from build123d import *

# Parameters (mm, degrees)
F0_W          = 465
F0_H          = 360
F1_DEPTH      = 82
F3_DEPTH      = 238.8411541644
F3_DEPTH_BACK = 251
F5_DEPTH      = 190
F5_DEPTH_BACK = 341
F6_T          = 18
F6_T3_DEPTH   = 370.2074342574
F6_T5_DEPTH   = 471


# Not quite as in the source:
# - a shell that OpenCascade refuses in one call is made with other operations: the cavity is built on its own and cut out


with BuildPart() as f1:
    # F0 (on Top) → F1 (new body)
    with BuildSketch(Plane.XY):
        with Locations((6.3401541644, 0)):
            Rectangle(F0_W, F0_H)
    extrude(amount=-F1_DEPTH)

    # F2 (on Right) → F3 (cut, two sides)
    with BuildSketch(Plane.YZ) as f3_sk:
        Polygon((-210, -15), (-210, -112), (-150, -112), (-167.1037171287, -15), align=None)
        Polygon((210, -15), (167.1037171287, -15), (150, -112), (210, -112), align=None)
    extrude(amount=F3_DEPTH, mode=Mode.SUBTRACT)
    extrude(f3_sk.sketch, amount=-F3_DEPTH_BACK, mode=Mode.SUBTRACT)

    # F4 (on Front) → F5 (cut, two sides)
    with BuildSketch(Plane.XZ) as f5_sk:
        Polygon((-241.1598458356, -15), (-241.1598458356, -185.1384545885), (-181.1598458356, -185.1384545885), (-211.1598458356, -15), align=None)
        Polygon((253.8401541644, -15), (223.8401541644, -15), (193.8816988413, -154.3605614963), (253.8401541644, -156.5929672103), align=None)
    extrude(amount=F5_DEPTH, mode=Mode.SUBTRACT)
    extrude(f5_sk.sketch, amount=-F5_DEPTH_BACK, mode=Mode.SUBTRACT)

    # F6: shell of thickness 18, made by hand


with BuildPart() as f6_core1:
    # F6_t2: copy of F1
    add(f1.part)

    # the walls: a layer under each face that stays
    f6_faces = [f6_core1.faces().sort_by_distance(p)[0] for p in [
        (-226.1598458356, 0, -7.5),
        (6.3401541644, -180, -7.5),
        (238.8401541644, 0, -7.5),
        (223.3401541644, 168, -15),
        (6.3401541644, 161.196763275, -48.5),
        (5.0455852734, 0, -82),
        (216.6386314197, 0, -48.5),
        (6.3401541644, -161.196763275, -48.5),
        (-205.2528919819, 0, -48.5),
        (6.3401541644, 180, -7.5),
    ]]
    thicken(f6_faces, amount=-F6_T, mode=Mode.SUBTRACT)

    # F6_s4 → F6_t3 (cut)
    with BuildSketch(Plane.XZ.offset(-185.1037171287)):
        Polygon((-211.3371112312, -15.211256672), (-211.1598458356, 3), (-196.0560524744, 3), (-193.4333062814, -11.874332802), align=None)
        Polygon((224.0161338598, -15.2178305009), (223.8401541644, 3), (209.2984141185, 3), (206.2421846213, -11.2169499127), align=None)
    extrude(amount=F6_T3_DEPTH, mode=Mode.SUBTRACT)

    # F6_s6 → F6_t5 (cut)
    with BuildSketch(Plane.YZ.offset(-229.1598458356)):
        Polygon((-167.2809825243, -15.211256672), (-167.1037171287, 3), (-151.9999237675, 3), (-149.3771775745, -11.874332802), align=None)
        Polygon((167.2809825243, -15.211256672), (167.1037171287, 3), (151.9999237675, 3), (149.3771775745, -11.874332802), align=None)
    extrude(amount=F6_T5_DEPTH, mode=Mode.SUBTRACT)


with BuildPart() as f1_1:
    add(f1.part)

    # what is left inside the walls is the cavity
    f6_cavity = [f6_core1.part.solids().sort_by_distance(p)[0] for p in [
        (6.563215, -50.490314, -0.18),
    ]]
    add(f6_cavity, mode=Mode.SUBTRACT)


solid = f1_1.part
The listing builds one solid part. Answer for the finished solid, in the listing's coordinates (mm). A direction names the side the tool comes from. Give positions to 0.01 mm unless a question says otherwise; leave off trailing zeros. Loops run counter-clockwise (first coordinate to the right, second up) from the corner with the lowest first, then second, coordinate; pieces in that order, holes last.
Item 1: A cutting plane is placed at C-C (z = -30). Give the vertices of the cut face in (x, y), then the cut area to 3 significant figures.
Derived:
outline: (-208.51, -164.46) - (220.62, -164.46) - (220.62, 164.46) - (-208.51, 164.46) - close; hole (-190.24, -146.18) - (202.2, -146.18) - (202.2, 146.18) - (-190.24, 146.18) - close
area: 26,400 mm2
Item 2: A cutting plane is placed at B-B (x = -79.5). Give the vertices of the cut face in (y, z), then the cut area to 3 significant figures.
Derived:
outline: (-180, -15) - (-167.1, -15) - (-155.29, -82) - (155.29, -82) - (167.1, -15) - (180, -15) - (180, 0) - (151.47, 0) - (140.19, -64) - (-140.19, -64) - (-151.47, 0) - (-180, 0) - close
area: 8,330 mm2
Item 3: Find the intervals of material crossed by line 1 along Z through (x, y) = (-101.5, 118); line 2 along Y through (x, z) = (42, -34.5); line 3 along Y through (x, z) = (-21, -60.5), in increasing order.
Derived:
line 1: z = -82 to -64
line 2: y = -163.67 to -145.39, 145.39 to 163.67
line 3: y = -159.08 to -140.8, 140.8 to 159.08
Item 4: A tool of negligible diameter and unlimited length cuts with its end or side. For faces 5 (the flat face through (7, 174, -15)), 6 (the flat face through (3, -157, 0)), from which of +Z, -Z, +X, -X, +Y, -Y can it reach the whole face along a straight path? Write none if from no direction.
Derived:
face 5: -Z
face 6: +Z, +X, -X, +Y, -Y
Item 5: Each of these flat-tipped pins is pushed along its axis until it touches: pin 1 Ø10 at (y, z) = (73.5, -48) entering from -X; pin 2 Ø1 at (x, z) = (-86.5, -36.5) entering from +Y; pin 3 Ø1.5 at (x, y) = (-156.5, -37) entering from +Z. Where does it stop, or does it pass through?
Derived:
pin 1: stops at x = -206.22
pin 2: stops at y = 163.4
pin 3: stops at z = -64
Item 6: A cutting plane is placed at D-D (z = -74). Give the vertices of the cut face in (x, y), then the cut area to 3 significant figures.
Derived:
outline: (-200.76, -156.7) - (211.16, -156.7) - (211.16, 156.7) - (-200.76, 156.7) - close
area: 129,000 mm2
Item 7: A cutting plane is placed at A-A (y = 52). Give the vertices of the cut face in (x, z), then the cut area to 3 significant figures.
Derived:
outline: (-226.16, -15) - (-211.16, -15) - (-199.35, -82) - (209.44, -82) - (223.84, -15) - (238.84, -15) - (238.84, 0) - (208.65, 0) - (194.9, -64) - (-184.24, -64) - (-195.53, 0) - (-226.16, 0) - close
area: 10,200 mm2
Item 8: Determine the mould class of faces 1 (the flat face through (3, 2, -64)), 2 (the flat face through (201.87, 2.12, -31.55)), 3 (the flat face through (-226.16, -3, -7)), 4 (the flat face through (9.39, 161.28, -48.03)) for opening direction X: +X half, -X half, draft (parallel to the pull), parting line (faces both ways), or undercut.
Derived:
face 1: undercut
face 2: undercut
face 3: -X half
face 4: draft
